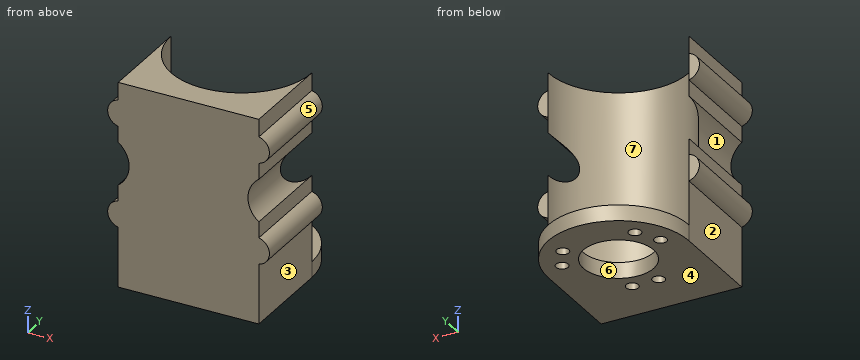
```python
from build123d import *

# Parameters (mm, degrees)
SKETCH3_W           = 40
SKETCH3_H           = 53.7
BOSS_EXTRUDE1_DEPTH = 27.5
BOSS_EXTRUDE4_DEPTH = 27.5
CUT_EXTRUDE1_DEPTH  = 28.5
SKETCH7_R           = 20
CUT_EXTRUDE2_DEPTH  = 54.7
BOSS_EXTRUDE5_DEPTH = 4.5
SKETCH9_R           = 10
CUT_EXTRUDE3_DEPTH  = 59.2000001
SKETCH10_R          = 1.75
CUT_EXTRUDE4_DEPTH  = 59.2000001


with BuildPart() as part:
    # Sketch3 → Boss-Extrude1 (new body)
    with BuildSketch(Plane(origin=(0, 0, 0), x_dir=(1, 0, 0), z_dir=(0, 1, 0))):
        with Locations((20, 26.85)):
            Rectangle(SKETCH3_W, SKETCH3_H)
    extrude(amount=BOSS_EXTRUDE1_DEPTH)

    # Sketch4 → Boss-Extrude4 (add)
    with BuildSketch(Plane(origin=(0, 27.5, 0), x_dir=(1, 0, 0), z_dir=(0, 1, 0))):
        with BuildLine():
            Line((0, 41.2), (0, 33.7))
            ThreePointArc((0, 33.7), (-2.999999474, 37.45), (0, 41.2))
        make_face()
        with BuildLine():
            Line((0, 12.5), (0, 5))
            ThreePointArc((0, 5), (-2.999999474, 8.75), (0, 12.5))
        make_face()
        with BuildLine():
            Line((40, 41.2), (40, 33.7))
            ThreePointArc((40, 33.7), (42.999999474, 37.45), (40, 41.2))
        make_face()
        with BuildLine():
            Line((40, 12.5), (40, 5))
            ThreePointArc((40, 5), (42.999999474, 8.75), (40, 12.5))
        make_face()
    extrude(amount=-BOSS_EXTRUDE4_DEPTH)

    # Sketch6 → Cut-Extrude1 (cut, through all)
    with BuildSketch(Plane(origin=(0, 27.5, 0), x_dir=(1, 0, 0), z_dir=(0, 1, 0))):
        with BuildLine():
            Line((0, 29.15), (0, 17.05))
            ThreePointArc((0, 17.05), (3.100001365, 23.1), (0, 29.15))
        make_face()
        with BuildLine():
            Line((40, 29.15), (40, 17.05))
            ThreePointArc((40, 17.05), (36.899998635, 23.1), (40, 29.15))
        make_face()
    extrude(amount=-CUT_EXTRUDE1_DEPTH, mode=Mode.SUBTRACT)

    # Sketch7 → Cut-Extrude2 (cut, through all)
    with BuildSketch(Plane(origin=(0, 0, -53.7), x_dir=(-1, 0, 0), z_dir=(0, 0, -1))):
        with Locations((-20, 27.5)):
            Circle(SKETCH7_R)
    extrude(amount=-CUT_EXTRUDE2_DEPTH, mode=Mode.SUBTRACT)

    # Sketch8 → Boss-Extrude5 (add)
    with BuildSketch(Plane(origin=(0, 0, -53.7), x_dir=(-1, 0, 0), z_dir=(0, 0, -1))):
        with BuildLine():
            Line((-40, 27.5), (-40, 0))
            Line((-40, 0), (0, 0))
            Line((0, 0), (0, 27.5))
            ThreePointArc((0, 27.5), (-20, 47.5), (-40, 27.5))
        make_face()
    extrude(amount=BOSS_EXTRUDE5_DEPTH)

    # Sketch9 → Cut-Extrude3 (cut, through all)
    with BuildSketch(Plane(origin=(0, 0, -58.2), x_dir=(-1, 0, 0), z_dir=(0, 0, -1))):
        with Locations((-20, 27.5)):
            Circle(SKETCH9_R)
    extrude(amount=-CUT_EXTRUDE3_DEPTH, mode=Mode.SUBTRACT)

    # Sketch10 → Cut-Extrude4 (cut, through all)
    with BuildSketch(Plane(origin=(0, 0, -58.2), x_dir=(-1, 0, 0), z_dir=(0, 0, -1))):
        with Locations((-23.75, 13.493305172)):
            Circle(SKETCH10_R)
        with Locations((-16.25, 13.493305172)):
            Circle(SKETCH10_R)
        with Locations((-34.005153544, 31.25575215)):
            Circle(SKETCH10_R)
        with Locations((-30.255153544, 37.750942678)):
            Circle(SKETCH10_R)
        with Locations((-9.744846456, 37.750942678)):
            Circle(SKETCH10_R)
        with Locations((-5.994846456, 31.25575215)):
            Circle(SKETCH10_R)
    extrude(amount=-CUT_EXTRUDE4_DEPTH, mode=Mode.SUBTRACT)


solid = part.part
```
Geometry check sheet. Reference: the model listing, model coordinates, mm. Face numbers are marked on the shaded views. A direction names the side the tool comes from. Give positions to 0.01 mm unless a question says otherwise; leave off trailing zeros. Write each loop counter-clockwise with the first axis right and the second up, starting at its lowest first coordinate (ties: lowest second). Pieces come first, ordered by that corner, then holes. Notation, with made-up numbers: (75.25, 3.25) - (88.25, 3.25) arc R21 cw to (88.25, 28.25) - close; hole circle Ø9 at (81.5, -22). An arc over 180 degrees is marked (long way). Use a Markdown table: item, result.
Q1. Section check D-D, the plane y = 9. Enter the section's corners in (x, z).
Computed:
| item | result |
|---|---|
| outline | (0, -58.2) - (40, -58.2) - (40, -41.2) arc R3.84 ccw to (40, -33.7) - (40, -29.15) arc R7.45 cw to (40, -17.05) - (40, -12.5) arc R3.84 ccw to (40, -5) - (40, 0) - (27.6, 0) - (27.6, -53.7) - (12.4, -53.7) - (12.4, 0) - (0, 0) - (0, -5) arc R3.84 ccw to (0, -12.5) - (0, -17.05) arc R7.45 cw to (0, -29.15) - (0, -33.7) arc R3.84 ccw to (0, -41.2) - close |
Q2. Set-up check for the marked faces 1, 2 and 3: record each of +Z, -Z, +X, -X, +Y, -Y from which the full face is reachable in a straight line by a thin tool's end or side.
Computed:
| item | result |
|---|---|
| face 1 | -X, +Y, -Y |
| face 2 | -Z, -X, +Y, -Y |
| face 3 | -Z, +X, +Y, -Y |
Q3. Go/stop test with flat-tipped pins: P1, Ø1.5, axis at x = -2, z = -7.5, coming from the +Y side; P2, Ø1.5, axis at x = 35, z = -46.5, coming from the -Y side; P3, Ø12, axis at x = 13, y = 30, coming from the +Z side; P4, Ø3.5, axis at y = 20, z = -14.5, coming from the +X side. Record where each tip stops, or that it passes through.
Computed:
| item | result |
|---|---|
| P1 | stops at y = 27.5 |
| P2 | stops at y = 0 |
| P3 | stops at z = -53.7 |
| P4 | stops at x = 40 |
Q4. Thickness scan on L1, parallel to Y at x = 16, z = -55; L2, parallel to Z at x = 7, y = 41.5; L3, parallel to Y at x = 32, z = -51. Record the ranges inside material, lowest first. Write a range as [from, to].
Computed:
| item | result |
|---|---|
| L1 | y = [0, 11.76], [15.23, 18.33], [36.67, 47.1] |
| L2 | z = [-58.2, -53.7] |
| L3 | y = [0, 11.5] |
Q5. Section check A-A, the plane x = 20. Enter the section's corners in (y, z), then the cut area to 4 significant figures.
Computed:
| item | result |
|---|---|
| outline | (0, -58.2) - (17.5, -58.2) - (17.5, -53.7) - (7.5, -53.7) - (7.5, 0) - (0, 0) - close; (37.5, -58.2) - (47.5, -58.2) - (47.5, -53.7) - (37.5, -53.7) - close |
| area | 526.5 mm² |
Q6. Draft check along X on the marked faces 4, 5, 6 and 7. Enter one of: pulls with the +X half, pulls with the -X half, needs draft (parallel to the pull), parting line crosses it, or undercut.
Computed:
| item | result |
|---|---|
| face 4 | needs draft |
| face 5 | pulls with the +X half |
| face 6 | undercut |
| face 7 | undercut |
Q7. Section check B-B, the plane y = 22. Enter the section's corners in (x, z), then the cut area to 3 significant figures.
Computed:
| item | result |
|---|---|
| outline | (0, -58.2) - (11.65, -58.2) - (11.65, -53.7) - (0.77, -53.7) - (0.77, -28.51) arc R7.45 cw to (0, -29.15) - (0, -33.7) arc R3.84 ccw to (0, -41.2) - close; (0, -17.05) arc R7.45 cw to (0.77, -17.69) - (0.77, 0) - (0, 0) - (0, -5) arc R3.84 ccw to (0, -12.5) - close; (28.35, -58.2) - (40, -58.2) - (40, -41.2) arc R3.84 ccw to (40, -33.7) - (40, -29.15) arc R7.45 cw to (39.23, -28.51) - (39.23, -53.7) - (28.35, -53.7) - close; (39.23, -17.69) arc R7.45 cw to (40, -17.05) - (40, -12.5) arc R3.84 ccw to (40, -5) - (40, 0) - (39.23, 0) - close |
| area | 237 mm² |
Q8. Section check C-C, the plane z = -52. Enter the section's corners in (x, y), then the cut area to 3 significant figures.
Computed:
| item | result |
|---|---|
| outline | (0, 0) - (40, 0) - (40, 27.5) arc R20 cw to (0, 27.5) - close |
| area | 472 mm² |
